Drawing for the job (mm, zero at the part's lowest x, y, z). Coordinates: 2 decimals unless noted, no trailing zeros. Loops run counter-clockwise (first coordinate to the right, second up) from the corner with the lowest first, then second, coordinate; pieces in that order, holes last. Notation, with made-up numbers: (-9.5, 69.5) - (-0.5, 69.5) arc R26 cw to (-0.5, 96.5) - close; hole circle Ø4 at (88, 39.5). An arc over 180 degrees is marked (long way). Put each result on its own line as item: value.
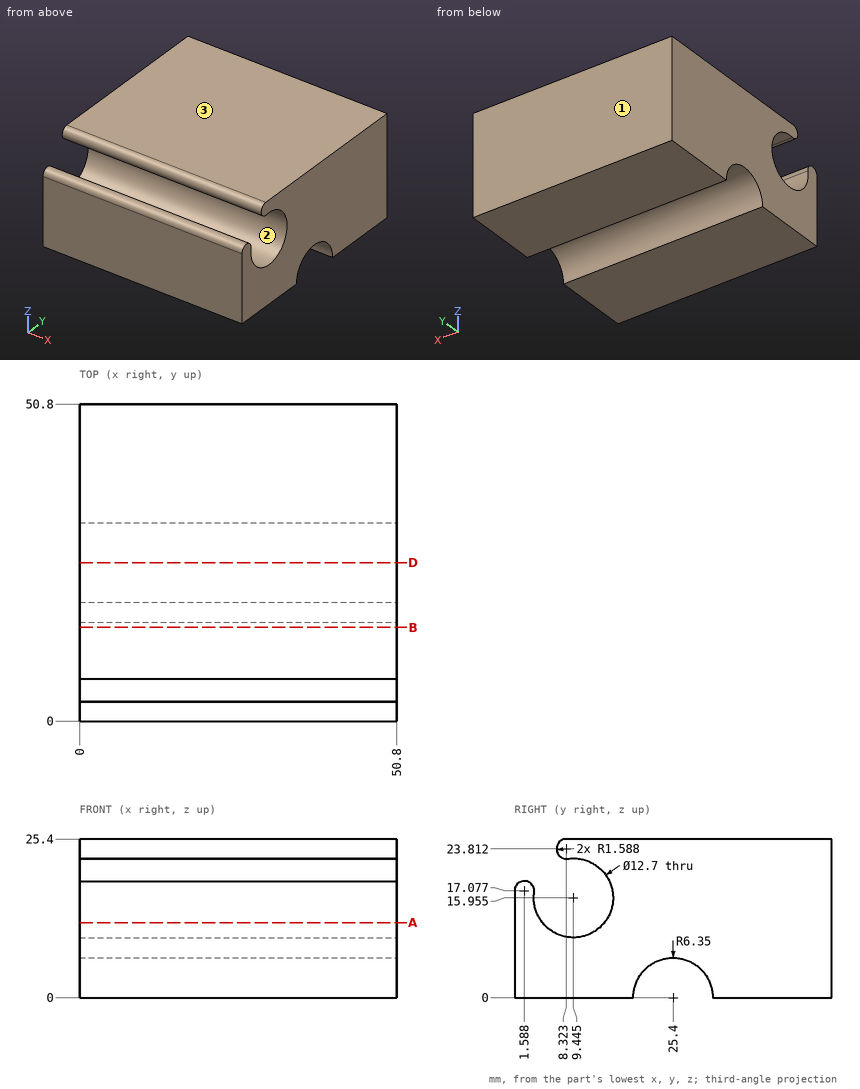
Q1. Slice it at A-A, the plane z = 12. Give the cut face in (x, y), then the cut area to 3 significant figures.
Determined:
outline: (0, 0) - (50.8, 0) - (50.8, 4.48) - (0, 4.48) - close; (0, 14.41) - (50.8, 14.41) - (50.8, 50.8) - (0, 50.8) - close
area: 2,080 mm2
Q2. Mould opens along Y. For the marked faces 1, 2 and 3 say: +Y half, -Y half, draft (parallel to the pull), parting line (faces both ways), or undercut.
Determined:
face 1: +Y half
face 2: undercut
face 3: draft
Q3. Slice it at D-D, the plane y = 25.4. Give the cut face in (x, z).
Determined:
outline: (0, 6.35) - (50.8, 6.35) - (50.8, 25.4) - (0, 25.4) - close
Q4. Slice it at B-B, the plane y = 15. Give the cut face in (x, z).
Determined:
outline: (0, 0) - (50.8, 0) - (50.8, 12.88) - (0, 12.88) - close; (0, 19.03) - (50.8, 19.03) - (50.8, 25.4) - (0, 25.4) - close
Q5. Wall check: L1, parallel to Z at x = 15, y = 9.5 (1 decimal); L2, parallel to Y at x = 32, z = 16.5; L3, parallel to Y at x = 14, z = 3.5. Give the ranges that are in metal, low to high. Write a range as from..to.
Determined:
L1: 0..9.6, 22.3..25.4
L2: 0..3.12, 15.77..50.8
L3: 0..20.1, 30.7..50.8
